```python
from build123d import *

# Parameters (mm, degrees)
BOSS_EXTRUDE1_DEPTH = 10
SKETCH2_R           = 4
CUT_EXTRUDE1_DEPTH  = 4.4
CUT_EXTRUDE2_REACH  = 23.339
SKETCH3_R           = 2.15
SKETCH4_R           = 7
CUT_EXTRUDE3_DEPTH  = 2
CUT_EXTRUDE4_REACH  = 24.091
SKETCH5_R           = 2.5
CUT_EXTRUDE5_START  = -2
SKETCH6_R           = 7
CUT_EXTRUDE5_DEPTH  = 2


with BuildPart() as part:
    # Sketch1 → Boss-Extrude1 (new body)
    with BuildSketch(Plane(origin=(0, 0, 0), x_dir=(1, 0, 0), z_dir=(0, 1, 0))):
        with BuildLine():
            Line((-10, 13), (-10, -13))
            ThreePointArc((-10, -13), (0, -18), (10, -13))
            Line((10, -13), (10, 13))
            ThreePointArc((10, 13), (0, 18), (-10, 13))
        make_face()
    extrude(amount=BOSS_EXTRUDE1_DEPTH)

    # Sketch2 → Cut-Extrude1 (cut)
    with BuildSketch(Plane(origin=(0, 10, 0), x_dir=(1, 0, 0), z_dir=(0, 1, 0))):
        with Locations(Location((0, 13, 0), (0, 0, 270))):
            Circle(SKETCH2_R)
        with Locations(Location((0, -13, 0), (0, 0, 270))):
            Circle(SKETCH2_R)
    extrude(amount=-CUT_EXTRUDE1_DEPTH, mode=Mode.SUBTRACT)

    # Sketch3 → Cut-Extrude2 (cut, up to next)
    with BuildSketch(Plane(origin=(0, 5.6, 0), x_dir=(1, 0, 0), z_dir=(0, 1, 0)), mode=Mode.PRIVATE) as cut_extrude2_sk1:
        with Locations(Location((0, 13, 0), (0, 0, 270))):
            Circle(SKETCH3_R)
    cut_extrude2_tool1 = extrude(cut_extrude2_sk1.sketch, amount=-CUT_EXTRUDE2_REACH, mode=Mode.PRIVATE) & part.part
    # Sketch3 → Cut-Extrude2 (cut, up to next)
    with BuildSketch(Plane(origin=(0, 5.6, 0), x_dir=(1, 0, 0), z_dir=(0, 1, 0)), mode=Mode.PRIVATE) as cut_extrude2_sk2:
        with Locations(Location((0, -13, 0), (0, 0, 270))):
            Circle(SKETCH3_R)
    cut_extrude2_tool2 = extrude(cut_extrude2_sk2.sketch, amount=-CUT_EXTRUDE2_REACH, mode=Mode.PRIVATE) & part.part
    add(cut_extrude2_tool1.solids().sort_by_distance((0, 5.6, -13))[0], mode=Mode.SUBTRACT)
    add(cut_extrude2_tool2.solids().sort_by_distance((0, 5.6, 13))[0], mode=Mode.SUBTRACT)

    # Sketch4 → Cut-Extrude3 (cut)
    with BuildSketch(Plane(origin=(0, 10, 0), x_dir=(1, 0, 0), z_dir=(0, 1, 0))):
        with Locations(Location((0, 0, 0), (0, 0, 270))):
            Circle(SKETCH4_R)
    extrude(amount=-CUT_EXTRUDE3_DEPTH, mode=Mode.SUBTRACT)

    # Sketch5 → Cut-Extrude4 (cut, up to next)
    with BuildSketch(Plane(origin=(0, 8, 0), x_dir=(1, 0, 0), z_dir=(0, 1, 0)), mode=Mode.PRIVATE) as cut_extrude4_sk1:
        with Locations(Location((0, 0, 0), (0, 0, 270))):
            Circle(SKETCH5_R)
    cut_extrude4_tool1 = extrude(cut_extrude4_sk1.sketch, amount=-CUT_EXTRUDE4_REACH, mode=Mode.PRIVATE) & part.part
    add(cut_extrude4_tool1.solids().sort_by_distance((0, 8, 0))[0], mode=Mode.SUBTRACT)

    # Sketch6 → Cut-Extrude5 (cut)
    with BuildSketch(Plane.XZ.offset(CUT_EXTRUDE5_START)):
        with Locations(Location((0, 0, 0), (0, 0, 90))):
            Circle(SKETCH6_R)
    extrude(amount=CUT_EXTRUDE5_DEPTH, mode=Mode.SUBTRACT)


solid = part.part
```
Could you check a few things on this model? Use its own coordinates, in mm. A direction names the side the tool comes from. Round coordinates to 2 decimals unless told otherwise and drop trailing zeros. Loops run counter-clockwise (first coordinate to the right, second up) from the corner with the lowest first, then second, coordinate; pieces in that order, holes last. Notation, with made-up numbers: M 66,81 L 83,81 A27 cw 83,104 Z; hole C 44.5,49 d5. An arc over 180 degrees is marked long. Write item = value, one per line.
1. Which directions (+Z, -Z, +X, -X, +Y, -Y) give clear straight access to the entire face, cutting with the end or side of a thin tool? Please do faces 4 (the face through (-6.834, 9.014, -1.517)), 5 (the face through (6.834, 1.014, -1.517)), 6 (the face through (0, 5, -18)).
Results below:
face_4 = +Y
face_5 = -Y
face_6 = -Z, +Y, -Y
2. I want a section at D-D, the plane x = -7.5. Write out the boundary of the cut face in (y, z).
Results below:
outline = M 0,-15.5 L 10,-15.5 L 10,15.5 L 0,15.5 Z
3. I want a section at A-A, the plane x = 0. Count the separate pieces of the cut face and the enclosed holes in it, and give its area (3 significant figures).
Results below:
separate_pieces = 4
enclosed_holes = 0
area = 155 mm²
4. Will these pins go through, and if not, where does the flat tip stop? P1, Ø2, axis at x = 1.5, y = 2.5, coming from the -Z side; P2, Ø2.5, axis at x = -2, z = -14, coming from the +Y side; P3, Ø3, axis at x = -6, y = 5.5, coming from the +Z side; P4, Ø3.5, axis at x = 0, z = -13, coming from the +Y side.
Results below:
P1 = -17.99
P2 = 5.6
P3 = 17.16
P4 = through
5. I want a section at C-C, the plane y = 2.5. Write out the boundary of the cut face in (x, z), and give its area (3 significant figures).
Results below:
outline = M -10,-13 A12.5 ccw 10,-13 L 10,13 A12.5 ccw -10,13 Z; hole C 0,0 d5; hole C 0,-13 d4.3; hole C 0,13 d4.3
area = 611 mm²
6. I need wall thicknesses on probe 1 along X at (y, z) = (6.8, 13); probe 2 along X at (y, z) = (9.55, 0); probe 3 along Z at (x, y) = (0.25, 7). Which ranges of each line are inside material? Lowest first, please.
Results below:
probe_1 = -10 to -4, 4 to 10
probe_2 = -10 to -7, 7 to 10
probe_3 = -18 to -16.99, -9.01 to -2.49, 2.49 to 9.01, 16.99 to 18
7. Thinking about a two-plate mould opening in X: for faces 1 (the face through (-2.44, 5.04, -0.54)), 2 (the face through (10, 5, 0)), 3 (the face through (0, 0, 8)), which applies, +X half, -X half, draft (parallel to the pull), parting line (faces both ways), or undercut?
Results below:
face_1 = undercut
face_2 = +X half
face_3 = draft
8. I want a section at B-B, the plane z = 0. Write out the boundary of the cut face in (x, y).
Results below:
outline = M -10,0 L -7,0 L -7,2 L -2.5,2 L -2.5,8 L -7,8 L -7,10 L -10,10 Z; M 2.5,2 L 7,2 L 7,0 L 10,0 L 10,10 L 7,10 L 7,8 L 2.5,8 Z
